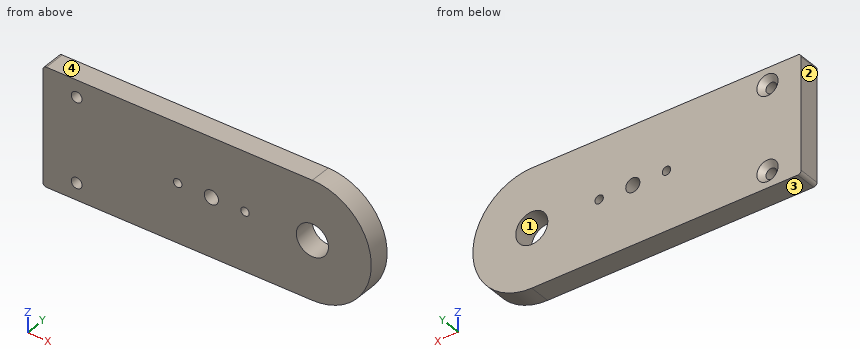
from build123d import *

# Parameters (mm, degrees)
SKETCH2_R                                       = 4.7625
BOSS_EXTRUDE1_DEPTH                             = 6.35
CSK_FOR_M3_FLAT_HEAD_MACHINE_SCREW1_D           = 3.2
CSK_FOR_M3_FLAT_HEAD_MACHINE_SCREW1_CSINK_D     = 6.3
CSK_FOR_M3_FLAT_HEAD_MACHINE_SCREW1_CSINK_ANGLE = 90
TAP_DRILL_FOR_M3X0_5_TAP1_D                     = 2.5
FILLET1_R                                       = 1
TAP_DRILL_FOR_M5X0_8_TAP1_D                     = 4.2


with BuildPart() as part:
    # Sketch2 → Boss-Extrude1 (new body)
    with BuildSketch(Plane(origin=(0, 0, 0), x_dir=(1, 0, 0), z_dir=(0, 1, 0))):
        with BuildLine():
            Line((70, 17.5), (-10, 17.5))
            Line((-10, 17.5), (-10, -17.5))
            Line((-10, -17.5), (70, -17.5))
            ThreePointArc((70, -17.5), (87.5, 0), (70, 17.5))
        make_face()
        with Locations((70, 0)):
            Circle(SKETCH2_R, mode=Mode.SUBTRACT)
    extrude(amount=-BOSS_EXTRUDE1_DEPTH)

    # CSK for M3 Flat Head Machine Screw1 (through all)
    with Locations(Plane(origin=(0, 0, -12.5), x_dir=(0, 0, 1), z_dir=(0, 1, 0))):
        with Locations((0, 0), (25, 0)):
            CounterSinkHole(CSK_FOR_M3_FLAT_HEAD_MACHINE_SCREW1_D / 2, CSK_FOR_M3_FLAT_HEAD_MACHINE_SCREW1_CSINK_D / 2, counter_sink_angle=CSK_FOR_M3_FLAT_HEAD_MACHINE_SCREW1_CSINK_ANGLE)

    # Tap Drill for M3x0.5 Tap1 (through all)
    with Locations(Plane(origin=(30, 0, 0), x_dir=(0, 0, 1), z_dir=(0, 1, 0))):
        with Locations((0, 0), (0, 20)):
            Hole(TAP_DRILL_FOR_M3X0_5_TAP1_D / 2)

    # Fillet1
    fillet1_edges = [part.edges().sort_by_distance(p)[0] for p in [
        (-10, -3.175, 17.5),
        (-10, -3.175, -17.5),
    ]]
    fillet(fillet1_edges, radius=FILLET1_R)

    # Tap Drill for M5x0.8 Tap1 (through all)
    with Locations(Plane(origin=(40, 0, 0), x_dir=(0, 0, 1), z_dir=(0, 1, 0))):
        with Locations((0, 0)):
            Hole(TAP_DRILL_FOR_M5X0_8_TAP1_D / 2)


solid = part.part
Work out the finished part from the listing and answer in its coordinate system (mm). Face numbers are marked on the shaded views. Give positions to 0.01 mm unless a question says otherwise; leave off trailing zeros. Order: outer loops, then holes, each group sorted by start corner. A loop starts at its lowest first (then second) coordinate and runs counter-clockwise, first axis right, second up. Notation, with made-up numbers: M 54.25,-4 L 86.25,-4 A15 ccw 86.25,6 Z; hole C -39,62 d6. An arc over 180 degrees is marked long. Return JSON: item names as keys, results as strings.
Q1. The mould has two halves that part along Z. Classify the marked faces 1, 2, 3 and 4: pulls with the +Z half, pulls with the -Z half, needs draft (parallel to the pull), parting line crosses it, or undercut.
Answer below:
{"face 1": "undercut", "face 2": "needs draft", "face 3": "pulls with the -Z half", "face 4": "pulls with the +Z half"}
Q2. Find section C-C, the plane z = 0. Write down the section's boundary in (x, y).
Answer below:
{"outline": "M -10,-6.35 L 28.75,-6.35 L 28.75,0 L -10,0 Z; M 31.25,-6.35 L 37.9,-6.35 L 37.9,0 L 31.25,0 Z; M 42.1,-6.35 L 48.75,-6.35 L 48.75,0 L 42.1,0 Z; M 51.25,-6.35 L 65.24,-6.35 L 65.24,0 L 51.25,0 Z; M 74.76,-6.35 L 87.5,-6.35 L 87.5,0 L 74.76,0 Z"}
Q3. Find section B-B, the plane x = 0. Write down the section's boundary in (y, z).
Answer below:
{"outline": "M -6.35,-17.5 L 0,-17.5 L 0,-15.65 L -1.55,-14.1 L -6.35,-14.1 Z; M -6.35,-10.9 L -1.55,-10.9 L 0,-9.35 L 0,9.35 L -1.55,10.9 L -6.35,10.9 Z; M -6.35,14.1 L -1.55,14.1 L 0,15.65 L 0,17.5 L -6.35,17.5 Z"}
Q4. Find section A-A, the plane y = -3.25. State how many separate pieces and enclosed holes the cut face has, and give its area (3 significant figures).
Answer below:
{"separate pieces": "1", "enclosed holes": "6", "area": "3,170 mm^2"}
Q5. Find section D-D, the plane x = 50. Write down the section's boundary in (y, z).
Answer below:
{"outline": "M -6.35,-17.5 L 0,-17.5 L 0,-1.25 L -6.35,-1.25 Z; M -6.35,1.25 L 0,1.25 L 0,17.5 L -6.35,17.5 Z"}
Q6. Each of these flat-tipped pins is pushed along its axis until it touches: pin 1 (8.5 mm diameter, centred on x = 70, z = 0, fed in from +Y); pin 2 (1.5 mm diameter, centred on y = -1.5, z = 2.5, fed in from +X); pin 3 (5 mm diameter, centred on x = 0, z = -12.5, fed in from +Y). Where does it stop, or does it pass through?
Answer below:
{"pin 1": "passes through", "pin 2": "stops at x = 87.41", "pin 3": "stops at y = -0.65"}
Q7. Find the intervals of material crossed by line 1 along X through (y, z) = (-1.5, 0); line 2 along Z through (x, y) = (0, -3.65); line 3 along Z through (x, y) = (70, -3.5), in increasing order. Write a range as [from, to].
Answer below:
{"line 1": "x = [-10, 28.75], [31.25, 37.9], [42.1, 48.75], [51.25, 65.24], [74.76, 87.5]", "line 2": "z = [-17.5, -14.1], [-10.9, 10.9], [14.1, 17.5]", "line 3": "z = [-17.5, -4.76], [4.76, 17.5]"}
